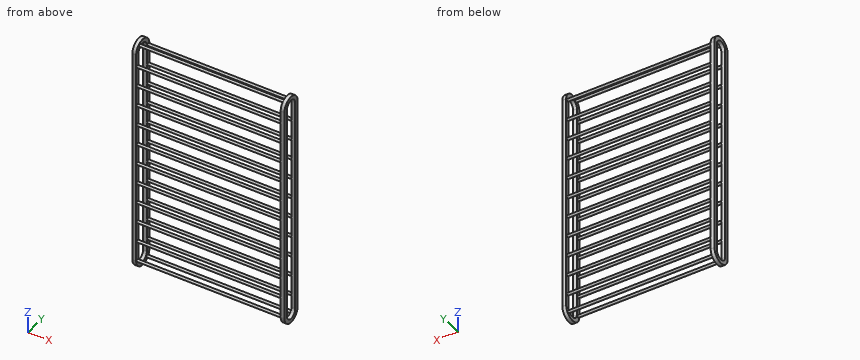
from build123d import *

# Parameters (mm, degrees)
SKETCH1_W           = 100
SKETCH1_H           = 100
BOSS_EXTRUDE1_DEPTH = 50
BOSS_EXTRUDE2_DEPTH = 30
SKETCH4_W           = 100
SKETCH4_H           = 30
BOSS_EXTRUDE3_DEPTH = 30
SKETCH5_W           = 50
SKETCH5_H           = 100
CUT_EXTRUDE1_DEPTH  = 110
LPATTERN1_COUNT     = 2
LPATTERN1_PITCH     = 1170
SKETCH6_R           = 10
BOSS_EXTRUDE4_DEPTH = 1160
LPATTERN2_COUNT     = 11
LPATTERN2_PITCH     = 160
SKETCH7_R           = 10
BOSS_EXTRUDE5_DEPTH = 1160
LPATTERN3_COUNT     = 11
LPATTERN3_PITCH     = 160
SKETCH8_R           = 10
BOSS_EXTRUDE6_DEPTH = 1160
SKETCH9_R           = 10
BOSS_EXTRUDE7_DEPTH = 1160


with BuildPart() as part:
    # Sketch1 → Boss-Extrude1 (new body)
    with BuildSketch(Plane(origin=(0, 0, 0), x_dir=(0, 0, -1), z_dir=(1, 0, 0))):
        with Locations((15.625, -21.033653846)):
            Rectangle(SKETCH1_W, SKETCH1_H)
    extrude(amount=BOSS_EXTRUDE1_DEPTH)



with BuildPart() as body_2:
    # Sketch3 → Boss-Extrude2 (new body)
    with BuildSketch(Plane(origin=(50, 0, 0), x_dir=(0, 0, -1), z_dir=(1, 0, 0))):
        with BuildLine():
            Line((-34.375, -13.682922568), (-34.375, 16.317077432))
            Line((-34.375, 16.317077432), (-746.477720281, 16.317077432))
            ThreePointArc((-746.477720281, 16.317077432), (-826.477720281, -63.682922568), (-746.477720281, -143.682922568))
            Line((-746.477720281, -143.682922568), (953.522279719, -143.682922568))
            ThreePointArc((953.522279719, -143.682922568), (1033.522279719, -63.682922568), (953.522279719, 16.317077432))
            Line((953.522279719, 16.317077432), (65.625, 16.317077432))
            Line((65.625, 16.317077432), (65.625, -13.682922568))
            Line((65.625, -13.682922568), (953.522279719, -13.682922568))
            ThreePointArc((953.522279719, -13.682922568), (1003.522279719, -63.682922568), (953.522279719, -113.682922568))
            Line((953.522279719, -113.682922568), (-746.477720281, -113.682922568))
            ThreePointArc((-746.477720281, -113.682922568), (-796.477720281, -63.682922568), (-746.477720281, -13.682922568))
            Line((-746.477720281, -13.682922568), (-34.375, -13.682922568))
        make_face()
    extrude(amount=BOSS_EXTRUDE2_DEPTH)


with BuildPart() as part_1:
    add(part.part)

    add(body_2.part)  # Boss-Extrude3 merges body 2
    # Sketch4 → Boss-Extrude3 (add)
    with BuildSketch(Plane(origin=(80, 0, 0), x_dir=(0, 0, -1), z_dir=(1, 0, 0))):
        with Locations((15.625, 1.317077432)):
            Rectangle(SKETCH4_W, SKETCH4_H)
    extrude(amount=-BOSS_EXTRUDE3_DEPTH)

    # Sketch5 → Cut-Extrude1 (cut)
    with BuildSketch(Plane(origin=(0, 28.966346154, 0), x_dir=(1, 0, 0), z_dir=(0, 1, 0))):
        with Locations((25, 15.625)):
            Rectangle(SKETCH5_W, SKETCH5_H)
    extrude(amount=-CUT_EXTRUDE1_DEPTH, mode=Mode.SUBTRACT)


with BuildPart() as lpattern1_1:
    # LPattern1: pattern copy
    add(part_1.part.moved(Location(Vector(1, 0, 0) * (1 * LPATTERN1_PITCH))))


with BuildPart() as part_2:
    add(part_1.part)

    add(lpattern1_1.part)  # Boss-Extrude4 merges LPattern1_1
    # Sketch6 → Boss-Extrude4 (add)
    with BuildSketch(Plane(origin=(80, 0, 0), x_dir=(0, 0, -1), z_dir=(1, 0, 0))):
        with Locations((-744.882973678, 0)):
            Circle(SKETCH6_R)
    boss_extrude4 = extrude(amount=BOSS_EXTRUDE4_DEPTH)

    # LPattern2: Boss-Extrude4 ×11
    with Locations(*[(0, 0, -i * LPATTERN2_PITCH) for i in range(1, LPATTERN2_COUNT)]):
        add(boss_extrude4)

    # Sketch7 → Boss-Extrude5 (add)
    with BuildSketch(Plane(origin=(80, 0, 0), x_dir=(0, 0, -1), z_dir=(1, 0, 0))):
        with Locations((956.928162623, -128.682922568)):
            Circle(SKETCH7_R)
    boss_extrude5 = extrude(amount=BOSS_EXTRUDE5_DEPTH)

    # LPattern3: Boss-Extrude5 ×11
    with Locations(*[(0, 0, i * LPATTERN3_PITCH) for i in range(1, LPATTERN3_COUNT)]):
        add(boss_extrude5)

    # Sketch8 → Boss-Extrude6 (add)
    with BuildSketch(Plane(origin=(80, 0, 0), x_dir=(0, 0, -1), z_dir=(1, 0, 0))):
        with Locations((-799.767519163, -100.901161848)):
            Circle(SKETCH8_R)
    extrude(amount=BOSS_EXTRUDE6_DEPTH)

    # Sketch9 → Boss-Extrude7 (add)
    with BuildSketch(Plane(origin=(80, 0, 0), x_dir=(0, 0, -1), z_dir=(1, 0, 0))):
        with Locations((992.567145138, -11.716601895)):
            Circle(SKETCH9_R)
    extrude(amount=BOSS_EXTRUDE7_DEPTH)


solid = part_2.part
For this review, take the finished solid that the model builds, in its own axes (mm). Round coordinates to 2 decimals unless told otherwise and drop trailing zeros. Loops run counter-clockwise (first coordinate to the right, second up) from the corner with the lowest first, then second, coordinate; pieces in that order, holes last. Notation, with made-up numbers: (87, 46.25) - (115, 46.25) arc R15 cw to (115, 59.25) - close; hole circle Ø11 at (-36, -26). An arc over 180 degrees is marked (long way). Use one line per item in the form item = value.
1) Clearance check with flat-ended pins moving along their axes: P1, Ø2, axis at x = 692, y = -22, coming from the +Z side; P2, Ø6, axis at x = 175, y = -124, coming from the -Z side; P3, Ø5, axis at x = 1014.5, y = -14, coming from the -Z side. State where each tip first meets the part, or that it passes through.
Solutions:
P1 = -988.85
P2 = -966.79
P3 = -1002.57
2) We need section B-B on x = 925. State how many separate pieces and enclosed holes the cut face has, then the cut area to 3 significant figures.
Solutions:
separate_pieces = 24
enclosed_holes = 0
area = 7,540 mm2
3) We need section A-A on y = -69. Write out the cut boundary in (x, z).
Solutions:
outline = (50, -1033.35) - (80, -1033.35) - (80, -1003.24) - (50, -1003.24) - close; (50, 796.19) - (80, 796.19) - (80, 826.3) - (50, 826.3) - close; (1220, -1033.35) - (1250, -1033.35) - (1250, -1003.24) - (1220, -1003.24) - close; (1220, 796.19) - (1250, 796.19) - (1250, 826.3) - (1220, 826.3) - close
4) Wall thickness on probe 1 along X at (y, z) = (-8, -316); probe 2 along Z at (x, y) = (832, -103); probe 3 along Y at (x, z) = (1091, 643): over which ranges is each line inside the solid? List them lowest first.
Solutions:
probe_1 = 50 to 80, 1220 to 1250
probe_2 = 789.99 to 809.54
probe_3 = -138.68 to -118.68
